from build123d import *

# Parameters (mm, degrees)
BOSS_EXTRUDE1_DEPTH = 20
SKETCH2_R           = 1.75
SKETCH2_R_2         = 2.25
BOSS_EXTRUDE2_DEPTH = 3
FILLET1_R           = 8
SKETCH3_W           = 60
SKETCH3_H           = 3
BOSS_EXTRUDE3_DEPTH = 65
FILLET2_R           = 15


with BuildPart() as part:
    # Sketch1 → Boss-Extrude1 (new body)
    with BuildSketch(Plane(origin=(0, 0, 0), x_dir=(1, 0, 0), z_dir=(0, 1, 0))):
        Polygon((-17.65, -1), (17.65, -1), (17.65, -14), (19.65, -14), (19.65, -1), (19.65, 1), (-19.65, 1), (-19.65, -1), (-19.65, -14), (-17.65, -14), align=None)
    extrude(amount=BOSS_EXTRUDE1_DEPTH)

    # Sketch2 → Boss-Extrude2 (add)
    with BuildSketch(Plane(origin=(0, 20, 0), x_dir=(1, 0, 0), z_dir=(0, 1, 0))):
        Polygon((-50, 1), (50, 1), (78.284271247, -27.284271247), (47.202085299, -58.366457196), (20, -31.164371897), (-15, -31.164371897), (-37.631017487, -53.795389384), (-71.213203436, -20.213203436), align=None)
        with Locations(Location((-61.850146281, -17.921214092, 0), (0, 0, 270))):
            Circle(SKETCH2_R, mode=Mode.SUBTRACT)
        with Locations(Location((-34.042532687, -42.328930623, 0), (0, 0, 270))):
            Circle(SKETCH2_R, mode=Mode.SUBTRACT)
        with Locations(Location((48.962338505, -48.018545271, 0), (0, 0, 270))):
            Circle(SKETCH2_R_2, mode=Mode.SUBTRACT)
        with Locations(Location((69.638225821, -28.478934535, 0), (0, 0, 90))):
            Circle(SKETCH2_R_2, mode=Mode.SUBTRACT)
        with Locations(Location((50.796458326, -8.541471766, 0), (0, 0, 270))):
            Circle(SKETCH2_R_2, mode=Mode.SUBTRACT)
        with Locations(Location((30.12057101, -28.081082501, 0), (0, 0, 90))):
            Circle(SKETCH2_R_2, mode=Mode.SUBTRACT)
    extrude(amount=BOSS_EXTRUDE2_DEPTH)

    # Fillet1
    fillet1_edges = [part.edges().sort_by_distance(p)[0] for p in [
        (-17.65, 20, 7.5),
        (0, 20, 1),
        (17.65, 20, 7.5),
    ]]
    fillet(fillet1_edges, radius=FILLET1_R)

    # Sketch3 → Boss-Extrude3 (add)
    with BuildSketch(Plane(origin=(0, 23, 0), x_dir=(1, 0, 0), z_dir=(0, 1, 0))):
        with Locations((2.5, -0.5)):
            Rectangle(SKETCH3_W, SKETCH3_H)
    extrude(amount=BOSS_EXTRUDE3_DEPTH)

    # Fillet2
    fillet2_edges = [part.edges().sort_by_distance(p)[0] for p in [
        (32.5, 23, 0.5),
        (-27.5, 23, 0.5),
    ]]
    fillet(fillet2_edges, radius=FILLET2_R)


solid = part.part
Input: part model. Units: mm. Frame: model coordinates. A direction names the side the tool comes from. Round coordinates to 2 decimals unless told otherwise and drop trailing zeros. Order: outer loops, then holes, each group sorted by start corner. A loop starts at its lowest first (then second) coordinate and runs counter-clockwise, first axis right, second up.
1. Set-up query: faces 4 (the face through (-18, 13, 14)), 5 (the face through (32.5, 63, 1)), 6 (the face through (2, 55, 2)), 7 (the face through (16.152, 16.66, 9.035)), 8 (the face through (-27.5, 63, 1)). Return all of +Z, -Z, +X, -X, +Y, -Y with unobstructed straight access to the full face (end or side cutting, diameter ignored); none if empty.
The answers:
face 4: +Z, +X, -X, -Y
face 5: +Z, -Z, +X, +Y
face 6: +Z, +X, -X, +Y
face 7: +Z, -Y
face 8: +Z, -Z, -X, +Y
2. Cut plane B-B, the plane x = -1.5. Output: boundary loops of the cut face in (y, z).
The answers:
outline: (0, -1) - (88, -1) - (88, 2) - (23, 2) - (23, 31.16) - (20, 31.16) - (20, 9) arc R8 cw to (12, 1) - (0, 1) - close
3. Cut plane A-A, the plane z = 35.5. Output: boundary loops of the cut face in (x, y).
The answers:
outline: (-55.93, 20) - (-19.34, 20) - (-19.34, 23) - (-55.93, 23) - close; (24.34, 20) - (70.07, 20) - (70.07, 23) - (24.34, 23) - close
4. Pin query (flat end, axial travel): P1, Ø2.5, axis at x = 30.12, z = 28.08, coming from the -Y side; P2, Ø12, axis at x = 2.5, z = 25, coming from the -Y side; P3, Ø12, axis at x = -13.5, y = 23.5, coming from the +Z side; P4, Ø1.5, axis at y = 71.5, z = 0.5, coming from the -X side. Return the tip coordinate at first contact, or that it passes through.
The answers:
P1: passes through
P2: stops at y = 20
P3: stops at z = 35.64
P4: stops at x = -27.5
5. Material intervals for line 1 (Y direction, x = 50.5, z = 22); line 2 (Z direction, x = 4.5, y = 75.5); line 3 (X direction, y = 21, z = 50.5), sorted ascending.
The answers:
line 1: y = 20 to 23
line 2: z = -1 to 2
line 3: x = -40.93 to -34.34, 39.34 to 55.07
6. Mould query, pull axis Z, two halves, no side actions, for faces 1 (the face through (0, 6, 1)), 2 (the face through (53.027, 21.479, 8.249)), 3 (the face through (64, 21, 13)). Classes: released by +Z, released by -Z, zero draft, split by the parting line, or undercut.
The answers:
face 1: released by +Z
face 2: undercut
face 3: released by -Z
7. Cut plane C-C, the plane z = 48. Output: boundary loops of the cut face in (x, y), then the cut area to 3 significant figures.
The answers:
outline: (-43.43, 20) - (-31.84, 20) - (-31.84, 23) - (-43.43, 23) - close; (36.84, 20) - (46.71, 20) - (46.71, 23) - (36.84, 23) - close; (51.21, 20) - (57.57, 20) - (57.57, 23) - (51.21, 23) - close
area: 83.5 mm2
8. Cut plane D-D, the plane y = 63. Output: boundary loops of the cut face in (x, z).
The answers:
outline: (-27.5, -1) - (32.5, -1) - (32.5, 2) - (-27.5, 2) - close
